The drawing under review shows one solid part. Ordinate dimensions are in mm from its lowest x, y, z. A direction names the side the tool comes from. Coordinates: 2 decimals unless noted, no trailing zeros. Order: outer loops, then holes, each group sorted by start corner. A loop starts at its lowest first (then second) coordinate and runs counter-clockwise, first axis right, second up. Notation, with made-up numbers: M -2,45 L 50,45 A19 cw 50,74 Z; hole C 16.25,6 d7. An arc over 180 degrees is marked long. Answer as a JSON object with one key per item and string values.
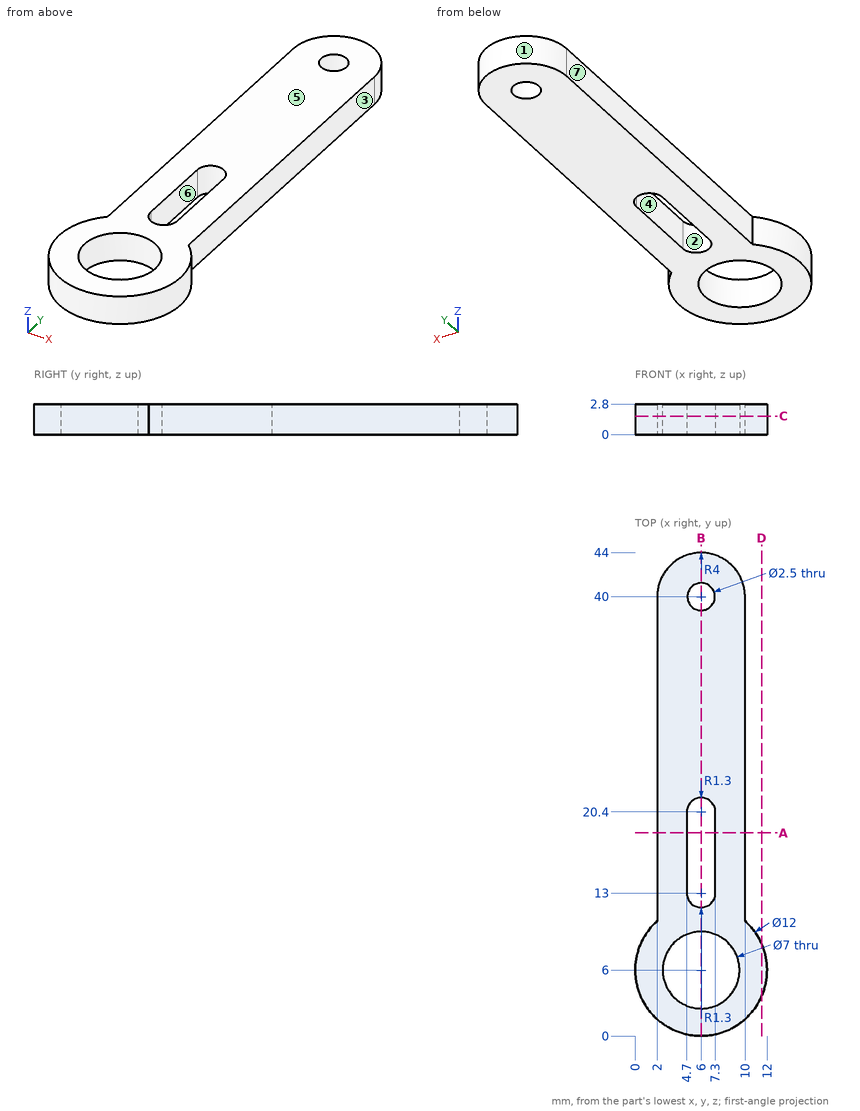
1) To check wall thickness, follow L1, parallel to Y at x = 6, z = 1.4; L2, parallel to X at y = 15, z = 0.5; L3, parallel to X at y = 31, z = 1.4. State the ranges of each line that lie inside material, in increasing order.
Taken from the geometry:
{"L1": "y = 0 to 2.5, 9.5 to 11.7, 21.7 to 38.75, 41.25 to 44", "L2": "x = 2 to 4.7, 7.3 to 10", "L3": "x = 2 to 10"}
2) Tool access review of the marked faces 5, 6 and 7: name each direction out of +Z, -Z, +X, -X, +Y, -Y from which nothing blocks a thin tool from reaching the whole face with its end or side.
Taken from the geometry:
{"face 5": "+Z, +X, -X, +Y, -Y", "face 6": "+Z, -Z", "face 7": "+Z, -Z, -X, +Y"}
3) Add section B-B (x = 6). State the section outline as (y, z) points.
Taken from the geometry:
{"outline": "M 0,0 L 2.5,0 L 2.5,2.8 L 0,2.8 Z; M 9.5,0 L 11.7,0 L 11.7,2.8 L 9.5,2.8 Z; M 21.7,0 L 38.75,0 L 38.75,2.8 L 21.7,2.8 Z; M 41.25,0 L 44,0 L 44,2.8 L 41.25,2.8 Z"}
4) Add section C-C (z = 1.7). State the section outline as (x, y) points.
Taken from the geometry:
{"outline": "M 2,10.47 A6 ccw long 10,10.47 L 10,40 A4 ccw 2,40 Z; hole C 6,6 d7; hole M 4.7,13 A1.3 ccw 7.3,13 L 7.3,20.4 A1.3 ccw 4.7,20.4 Z; hole C 6,40 d2.5"}
5) Add section D-D (x = 11.5). State the section outline as (y, z) points.
Taken from the geometry:
{"outline": "M 3.6,0 L 8.4,0 L 8.4,2.8 L 3.6,2.8 Z"}
6) Mouldability with a two-part tool opening along Y and no side actions: class the marked faces 1, 2, 3 and 4 as released by +Y, released by -Y, zero draft, split by the parting line, or undercut.
Taken from the geometry:
{"face 1": "released by +Y", "face 2": "undercut", "face 3": "zero draft", "face 4": "undercut"}
7) Add section A-A (y = 18.5). State the section outline as (x, z) points.
Taken from the geometry:
{"outline": "M 2,0 L 4.7,0 L 4.7,2.8 L 2,2.8 Z; M 7.3,0 L 10,0 L 10,2.8 L 7.3,2.8 Z"}
8) Insertion check: pin 1 Ø3 at (x, y) = (4, 29) entering from -Z; pin 2 Ø0.8 at (y, z) = (16, 1) entering from +X; pin 3 Ø1 at (y, z) = (16.5, 1) entering from -X; pin 4 Ø1.5 at (x, y) = (6, 40) entering from -Z. Each pin has a flat end and moves straight along its axis. Give the tip position at first contact, or say it passes through.
Taken from the geometry:
{"pin 1": "stops at z = 0", "pin 2": "stops at x = 10", "pin 3": "stops at x = 2", "pin 4": "passes through"}
